Here's how the part is built. I have some questions about the finished solid (model axes, mm). Coordinates: 2 decimals unless noted, no trailing zeros. Write each loop counter-clockwise with the first axis right and the second up, starting at its lowest first coordinate (ties: lowest second). Pieces come first, ordered by that corner, then holes.
(1) For pin 1 Ø1.5 at (y, z) = (198.5, 18) entering from +X; pin 2 Ø12 at (x, z) = (-58.5, -1.5) entering from +Y; pin 3 Ø8 at (x, z) = (376, -9.5) entering from -Y, each with a flat end and sliding along its axis, tell me the tip position at first contact or that it passes through.
(2) Imagine slicing it at A-A, the plane y = 0. List the corners of the cut face in (x, z) for me, plus the area to 3 significant figures.
(3) Imagine slicing it at B-B, the plane z = 9. List the corners of the cut face in (x, y) for me, plus the area to 3 significant figures.
(4) Imagine slicing it at C-C, the plane x = -315.5. State how many separate pieces and enclosed holes the cut face has, plus the area to 3 significant figures.
(5) Please list where these lines run through material, in increasing order: probe 1 along X at (y, z) = (0, -7); probe 2 along Y at (x, z) = (-131.5, -12); probe 3 along X at (y, z) = (375, -12).
```python
from build123d import *

# Parameters (mm, degrees)
CUT_EXTRUDE1_DEPTH = 127
SKETCH3_R          = 6.35
CUT_EXTRUDE2_DEPTH = 127


with BuildPart() as part:
    # Sketch1 → Revolve1 (revolve)
    with BuildSketch(Plane(origin=(0, 0, 0), x_dir=(1, 0, 0), z_dir=(0, 1, 0))):
        Polygon((0, 27.715882353), (0, -35.784117647), (-533.4, 11.43), (-533.4, 27.715882353), align=None)
    revolve(axis=Axis((38.1, 0, -15.015882353), (0, 0, 1)))

    # Sketch2 → Cut-Extrude1 (cut)
    with BuildSketch(Plane(origin=(0, 0, -27.715882353), x_dir=(-1, 0, 0), z_dir=(0, 0, -1))):
        with BuildLine():
            ThreePointArc((-85.306443453, -19.836041494), (-89.304656484, 0), (-85.306443453, 19.836041494))
            Line((-85.306443453, 19.836041494), (-514.216095648, 267.467144646))
            ThreePointArc((-514.216095648, 267.467144646), (-584.2, 0), (-514.216095648, -267.467144646))
            Line((-514.216095648, -267.467144646), (-85.306443453, -19.836041494))
        make_face()
        with BuildLine():
            ThreePointArc((-78.881737571, 30.963958506), (-63.702328242, 44.344533307), (-44.524705882, 50.8))
            Line((-44.524705882, 50.8), (-44.524705882, 546.062206305))
            ThreePointArc((-44.524705882, 546.062206305), (-311.15, 472.936473007), (-507.791389765, 278.595061658))
            Line((-507.791389765, 278.595061658), (-78.881737571, 30.963958506))
        make_face()
        with BuildLine():
            Line((-31.675294118, 546.062206305), (-31.675294118, 50.8))
            ThreePointArc((-31.675294118, 50.8), (-12.497671758, 44.344533307), (2.681737571, 30.963958506))
            Line((2.681737571, 30.963958506), (431.591389765, 278.595061658))
            ThreePointArc((431.591389765, 278.595061658), (234.95, 472.936473007), (-31.675294118, 546.062206305))
        make_face()
        with BuildLine():
            ThreePointArc((9.106443453, 19.836041494), (13.104656484, 0), (9.106443453, -19.836041494))
            Line((9.106443453, -19.836041494), (438.016095648, -267.467144646))
            ThreePointArc((438.016095648, -267.467144646), (508, 0), (438.016095648, 267.467144646))
            Line((438.016095648, 267.467144646), (9.106443453, 19.836041494))
        make_face()
        with BuildLine():
            ThreePointArc((2.681737571, -30.963958506), (-12.497671758, -44.344533307), (-31.675294118, -50.8))
            Line((-31.675294118, -50.8), (-31.675294118, -546.062206305))
            ThreePointArc((-31.675294118, -546.062206305), (234.95, -472.936473007), (431.591389765, -278.595061658))
            Line((431.591389765, -278.595061658), (2.681737571, -30.963958506))
        make_face()
        with BuildLine():
            ThreePointArc((-44.524705882, -50.8), (-63.702328242, -44.344533307), (-78.881737571, -30.963958506))
            Line((-78.881737571, -30.963958506), (-507.791389765, -278.595061658))
            ThreePointArc((-507.791389765, -278.595061658), (-311.15, -472.936473007), (-44.524705882, -546.062206305))
            Line((-44.524705882, -546.062206305), (-44.524705882, -50.8))
        make_face()
    extrude(amount=-CUT_EXTRUDE1_DEPTH, mode=Mode.SUBTRACT)

    # Sketch3 → Cut-Extrude2 (cut)
    with BuildSketch(Plane.XY):
        with Locations((982.963055161, 544.767048731)):
            Circle(SKETCH3_R)
        with Locations((963.263630927, -578.887452386)):
            Circle(SKETCH3_R)
        with Locations((-19.699424235, -1123.654501117)):
            Circle(SKETCH3_R)
        with Locations((-982.963055161, -544.767048731)):
            Circle(SKETCH3_R)
        with Locations((-963.263630927, 578.887452386)):
            Circle(SKETCH3_R)
        with Locations((19.699424235, 1123.654501117)):
            Circle(SKETCH3_R)
    extrude(amount=-CUT_EXTRUDE2_DEPTH, mode=Mode.SUBTRACT)


solid = part.part
```
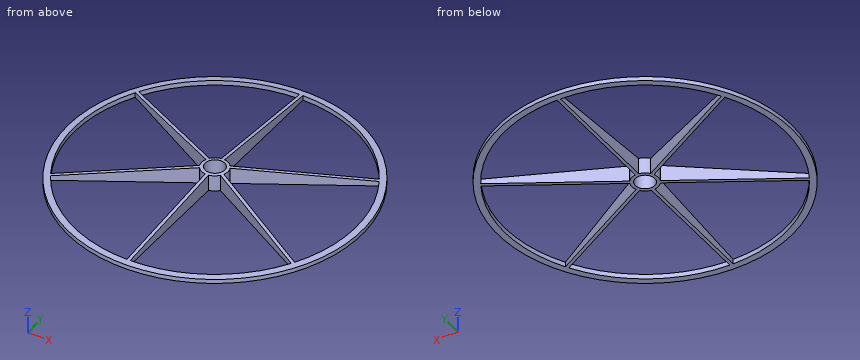
Recorded:
1. pin 1: stops at x = 44.52
1. pin 2: stops at y = 66.65
1. pin 3: stops at y = -463.46
2. outline: (-533.4, -27.72) - (-508, -27.72) - (-508, -9.18) - (-533.4, -11.43) - close; (-13.1, -27.72) - (0, -27.72) - (0, 35.78) - (-13.1, 34.62) - close; (76.2, -27.72) - (89.3, -27.72) - (89.3, 34.62) - (76.2, 35.78) - close; (584.2, -27.72) - (609.6, -27.72) - (609.6, -11.43) - (584.2, -9.18) - close
2. area: 2,530 mm2
3. outline: (-260.11, -164.75) arc R340.69 ccw to (-253.68, -175.88) - (-2.68, -30.96) arc R51.2 ccw to (31.68, -50.8) - (31.68, -340.63) arc R340.69 ccw to (44.52, -340.63) - (44.52, -50.8) arc R51.2 ccw to (78.88, -30.96) - (329.88, -175.88) arc R340.69 ccw to (336.31, -164.75) - (85.31, -19.84) arc R51.2 ccw to (85.31, 19.84) - (336.31, 164.75) arc R340.69 ccw to (329.88, 175.88) - (78.88, 30.96) arc R51.2 ccw to (44.52, 50.8) - (44.52, 340.63) arc R340.69 ccw to (31.68, 340.63) - (31.68, 50.8) arc R51.2 ccw to (-2.68, 30.96) - (-253.68, 175.88) arc R340.69 ccw to (-260.11, 164.75) - (-9.11, 19.84) arc R51.2 ccw to (-9.11, -19.84) - close; hole circle Ø76.2 at (38.1, 0)
3. area: 26,000 mm2
4. separate pieces: 4
4. enclosed holes: 0
4. area: 2,050 mm2
5. probe 1: x = -13.1 to 0, 76.2 to 89.3
5. probe 2: y = -545.75 to -519.1, -105.34 to -90.5, 90.5 to 105.34, 519.1 to 545.75
5. probe 3: x = -393.16 to -358.89, 31.68 to 44.52, 435.09 to 469.36
